```python
from build123d import *

# Parameters (mm, degrees)
ESQUISSE1_W            = 30
ESQUISSE1_H            = 30
BASE_PLATE_DEPTH       = 2
SKETCH_PERFORATIONS_R  = 0.5
CUT_PERFORATIONS_DEPTH = 10


with BuildPart() as part:
    # Esquisse1 → Base_Plate (new body)
    with BuildSketch(Plane.XY):
        Rectangle(ESQUISSE1_W, ESQUISSE1_H)
    extrude(amount=BASE_PLATE_DEPTH)

    # Sketch_Perforations → Cut_Perforations (cut)
    with BuildSketch(Plane.XY.offset(2)):
        with Locations((-3.1, -10.11)):
            Circle(SKETCH_PERFORATIONS_R)
        with Locations((-3.1, -7.22)):
            Circle(SKETCH_PERFORATIONS_R)
        with Locations((-3.1, -4.33)):
            Circle(SKETCH_PERFORATIONS_R)
        with Locations((-3.1, -1.44)):
            Circle(SKETCH_PERFORATIONS_R)
        with Locations((-3.1, 1.44)):
            Circle(SKETCH_PERFORATIONS_R)
        with Locations((-3.1, 4.33)):
            Circle(SKETCH_PERFORATIONS_R)
        with Locations((-3.1, 7.22)):
            Circle(SKETCH_PERFORATIONS_R)
        with Locations((-3.1, 10.11)):
            Circle(SKETCH_PERFORATIONS_R)
        with Locations((-1.03, -10.11)):
            Circle(SKETCH_PERFORATIONS_R)
        with Locations((-1.03, -7.22)):
            Circle(SKETCH_PERFORATIONS_R)
        with Locations((-1.03, -4.33)):
            Circle(SKETCH_PERFORATIONS_R)
        with Locations((-1.03, -1.44)):
            Circle(SKETCH_PERFORATIONS_R)
        with Locations((-1.03, 1.44)):
            Circle(SKETCH_PERFORATIONS_R)
        with Locations((-1.03, 4.33)):
            Circle(SKETCH_PERFORATIONS_R)
        with Locations((-1.03, 7.22)):
            Circle(SKETCH_PERFORATIONS_R)
        with Locations((-1.03, 10.11)):
            Circle(SKETCH_PERFORATIONS_R)
        with Locations((1.03, -10.11)):
            Circle(SKETCH_PERFORATIONS_R)
        with Locations((1.03, -7.22)):
            Circle(SKETCH_PERFORATIONS_R)
        with Locations((1.03, -4.33)):
            Circle(SKETCH_PERFORATIONS_R)
        with Locations((1.03, -1.44)):
            Circle(SKETCH_PERFORATIONS_R)
        with Locations((1.03, 1.44)):
            Circle(SKETCH_PERFORATIONS_R)
        with Locations((1.03, 4.33)):
            Circle(SKETCH_PERFORATIONS_R)
        with Locations((1.03, 7.22)):
            Circle(SKETCH_PERFORATIONS_R)
        with Locations((1.03, 10.11)):
            Circle(SKETCH_PERFORATIONS_R)
        with Locations((3.1, -10.11)):
            Circle(SKETCH_PERFORATIONS_R)
        with Locations((3.1, -7.22)):
            Circle(SKETCH_PERFORATIONS_R)
        with Locations((3.1, -4.33)):
            Circle(SKETCH_PERFORATIONS_R)
        with Locations((3.1, -1.44)):
            Circle(SKETCH_PERFORATIONS_R)
        with Locations((3.1, 1.44)):
            Circle(SKETCH_PERFORATIONS_R)
        with Locations((3.1, 4.33)):
            Circle(SKETCH_PERFORATIONS_R)
        with Locations((3.1, 7.22)):
            Circle(SKETCH_PERFORATIONS_R)
        with Locations((3.1, 10.11)):
            Circle(SKETCH_PERFORATIONS_R)
    extrude(amount=-CUT_PERFORATIONS_DEPTH, mode=Mode.SUBTRACT)


solid = part.part
```
Can you work these out from the model? Positions are in its coordinate system, mm. Coordinates: 2 decimals unless noted, no trailing zeros. Write each loop counter-clockwise with the first axis right and the second up, starting at its lowest first coordinate (ties: lowest second). Pieces come first, ordered by that corner, then holes. Notation, with made-up numbers: (65.25, 35) - (124.25, 35) arc R27 cw to (124.25, 54) - close; hole circle Ø9 at (78, 57.5). An arc over 180 degrees is marked (long way). Return JSON: item names as keys, results as strings.
Q1. Please list where this line runs through material, in increasing order: L1, parallel to X at y = 1.75, z = 0.8. Write a range as from..to.
Computed values:
{"L1": "x = -15..-3.49, -2.71..-1.42, -0.64..0.64, 1.42..2.71, 3.49..15"}
Q2. If we section it at A-A (y = 7.22): Please give me the cut outline in (x, z), then the cut area to 3 significant figures.
Computed values:
{"outline": "(-15, 0) - (-3.6, 0) - (-3.6, 2) - (-15, 2) - close; (-2.6, 0) - (-1.53, 0) - (-1.53, 2) - (-2.6, 2) - close; (-0.53, 0) - (0.53, 0) - (0.53, 2) - (-0.53, 2) - close; (1.53, 0) - (2.6, 0) - (2.6, 2) - (1.53, 2) - close; (3.6, 0) - (15, 0) - (15, 2) - (3.6, 2) - close", "area": "52.0 mm2"}
Q3. Thinking about a two-plate mould opening in Y: for faces 1 (the flat face through (0, -15, 1)), 2 (the cylindrical face through (0.965, -9.614, 1.014)), 3 (the flat face through (0, 0, 2)), which applies, +Y half, -Y half, draft (parallel to the pull), parting line (faces both ways), or undercut?
Computed values:
{"face 1": "-Y half", "face 2": "undercut", "face 3": "draft"}
Q4. If we section it at B-B (x = 1.03): Count the separate pieces of the cut face and the enclosed holes in it, then the cut area to 3 significant figures.
Computed values:
{"separate pieces": "9", "enclosed holes": "0", "area": "44.0 mm2"}
